```python
from build123d import *
from build123d.topology import SkipClean

# Parameters (mm, degrees)
BOSS_EXTRUDE1_DEPTH = 15
CUT_EXTRUDE1_DEPTH  = 5
BOSS_EXTRUDE2_DEPTH = 5
SKETCH3_R           = 15
CUT_EXTRUDE2_DEPTH  = 10


with BuildPart() as part:
    # Sketch1 → Boss-Extrude1 (new, symmetric)
    with BuildSketch(Plane.XY):
        with BuildLine():
            Line((-12.310096913, 2.170602221), (12.310096913, 2.170602221))
            ThreePointArc((12.310096913, 2.170602221), (0, -12.5), (-12.310096913, 2.170602221))
        make_face()
        with BuildLine():
            ThreePointArc((12.310096913, 2.170602221), (0, 12.5), (-12.310096913, 2.170602221))
            Line((-12.310096913, 2.170602221), (12.310096913, 2.170602221))
        make_face()
        with BuildLine():
            ThreePointArc((-12.310096913, 2.170602221), (0, -12.5), (12.310096913, 2.170602221))
            Line((12.310096913, 2.170602221), (15.337737359, -15))
            Line((15.337737359, -15), (-15.337737359, -15))
            Line((-15.337737359, -15), (-12.310096913, 2.170602221))
        make_face()
    extrude(amount=BOSS_EXTRUDE1_DEPTH, both=True)

    # Sketch1<3> → Cut-Extrude1 (cut, symmetric)
    with SkipClean():  # the faces are left unmerged after this step: merging them gives an invalid solid
        with BuildSketch(Plane.XY):
            with BuildLine():
                ThreePointArc((12.310096913, 2.170602221), (0, 12.5), (-12.310096913, 2.170602221))
                Line((-12.310096913, 2.170602221), (12.310096913, 2.170602221))
            make_face()
            with BuildLine():
                Line((-12.310096913, 2.170602221), (12.310096913, 2.170602221))
                ThreePointArc((12.310096913, 2.170602221), (0, -12.5), (-12.310096913, 2.170602221))
            make_face()
        extrude(amount=CUT_EXTRUDE1_DEPTH, both=True, mode=Mode.SUBTRACT)

    # Sketch2 → Boss-Extrude2 (add)
    with BuildSketch(Plane.XZ.offset(15)):
        with BuildLine():
            Line((-50, -7.5), (-23.848480035, -7.5))
            ThreePointArc((-23.848480035, -7.5), (-25, 0), (-23.848480035, 7.5))
            Line((-23.848480035, 7.5), (-50, 7.5))
            ThreePointArc((-50, 7.5), (-57.5, 0), (-50, -7.5))
        make_face()
        with BuildLine():
            Line((-23.848480035, -7.5), (-15.337737359, -7.5))
            Line((-15.337737359, -7.5), (-15.337737359, 7.5))
            Line((-15.337737359, 7.5), (-23.848480035, 7.5))
            ThreePointArc((-23.848480035, 7.5), (-25, 0), (-23.848480035, -7.5))
        make_face()
        with BuildLine():
            Line((-23.848480035, 7.5), (-15.337737359, 7.5))
            Line((-15.337737359, 7.5), (-15.337737359, 15))
            Line((-15.337737359, 15), (0, 15))
            Line((0, 15), (5.429049489, 24.403389552))
            ThreePointArc((5.429049489, 24.403389552), (-12.5, 21.650635095), (-23.848480035, 7.5))
        make_face()
        with BuildLine():
            ThreePointArc((5.429049489, 24.403389552), (12.5, 21.650635095), (18.419430546, 16.903389552))
            Line((18.419430546, 16.903389552), (31.495190528, 39.551270189))
            ThreePointArc((31.495190528, 39.551270189), (28.75, 49.796460718), (18.504809472, 47.051270189))
            Line((18.504809472, 47.051270189), (5.429049489, 24.403389552))
        make_face()
        with BuildLine():
            Line((15.337737359, 15), (15.337737359, 11.565740379))
            Line((15.337737359, 11.565740379), (18.419430546, 16.903389552))
            ThreePointArc((18.419430546, 16.903389552), (12.5, 21.650635095), (5.429049489, 24.403389552))
            Line((5.429049489, 24.403389552), (0, 15))
            Line((0, 15), (15.337737359, 15))
        make_face()
        with BuildLine():
            Line((18.419430546, 16.903389552), (15.337737359, 11.565740379))
            Line((15.337737359, 11.565740379), (15.337737359, -11.565740379))
            Line((15.337737359, -11.565740379), (18.419430546, -16.903389552))
            ThreePointArc((18.419430546, -16.903389552), (23.296842744, -9.069571003), (25, 0))
            ThreePointArc((25, 0), (23.296842744, 9.069571003), (18.419430546, 16.903389552))
        make_face()
        with BuildLine():
            ThreePointArc((6.495190528, -3.75), (3.75, -6.495190528), (0, -7.5))
            Line((0, -7.5), (-4.330127019, -7.5))
            Line((-4.330127019, -7.5), (0, -15))
            Line((0, -15), (15.337737359, -15))
            Line((15.337737359, -15), (15.337737359, -11.565740379))
            Line((15.337737359, -11.565740379), (8.660254038, 0))
            Line((8.660254038, 0), (6.495190528, -3.75))
        make_face()
        with BuildLine():
            Line((15.337737359, -15), (0, -15))
            Line((0, -15), (5.429049489, -24.403389552))
            ThreePointArc((5.429049489, -24.403389552), (12.5, -21.650635095), (18.419430546, -16.903389552))
            Line((18.419430546, -16.903389552), (15.337737359, -11.565740379))
            Line((15.337737359, -11.565740379), (15.337737359, -15))
        make_face()
        with BuildLine():
            ThreePointArc((18.419430546, -16.903389552), (12.5, -21.650635095), (5.429049489, -24.403389552))
            Line((5.429049489, -24.403389552), (18.504809472, -47.051270189))
            ThreePointArc((18.504809472, -47.051270189), (28.75, -49.796460718), (31.495190528, -39.551270189))
            Line((31.495190528, -39.551270189), (18.419430546, -16.903389552))
        make_face()
        with BuildLine():
            Line((-15.337737359, -15), (-15.337737359, -7.5))
            Line((-15.337737359, -7.5), (-23.848480035, -7.5))
            ThreePointArc((-23.848480035, -7.5), (-12.5, -21.650635095), (5.429049489, -24.403389552))
            Line((5.429049489, -24.403389552), (0, -15))
            Line((0, -15), (-15.337737359, -15))
        make_face()
        Polygon((0, -15), (-4.330127019, -7.5), (-15.337737359, -7.5), (-15.337737359, -15), align=None)
        with BuildLine():
            Line((-15.337737359, -7.5), (-4.330127019, -7.5))
            Line((-4.330127019, -7.5), (-6.495190528, -3.75))
            ThreePointArc((-6.495190528, -3.75), (-7.5, 0), (-6.495190528, 3.75))
            Line((-6.495190528, 3.75), (-4.330127019, 7.5))
            Line((-4.330127019, 7.5), (-15.337737359, 7.5))
            Line((-15.337737359, 7.5), (-15.337737359, -7.5))
        make_face()
        Polygon((-15.337737359, 15), (-15.337737359, 7.5), (-4.330127019, 7.5), (0, 15), align=None)
        with BuildLine():
            Line((6.495190528, 3.75), (8.660254038, 0))
            Line((8.660254038, 0), (15.337737359, 11.565740379))
            Line((15.337737359, 11.565740379), (15.337737359, 15))
            Line((15.337737359, 15), (0, 15))
            Line((0, 15), (-4.330127019, 7.5))
            Line((-4.330127019, 7.5), (0, 7.5))
            ThreePointArc((0, 7.5), (3.75, 6.495190528), (6.495190528, 3.75))
        make_face()
        Polygon((15.337737359, 11.565740379), (8.660254038, 0), (15.337737359, -11.565740379), align=None)
        with BuildLine():
            ThreePointArc((6.495190528, 3.75), (7.5, 0), (6.495190528, -3.75))
            Line((6.495190528, -3.75), (8.660254038, 0))
            Line((8.660254038, 0), (6.495190528, 3.75))
        make_face()
        with BuildLine():
            ThreePointArc((-6.495190528, -3.75), (-3.75, -6.495190528), (0, -7.5))
            ThreePointArc((0, -7.5), (3.75, -6.495190528), (6.495190528, -3.75))
            ThreePointArc((6.495190528, -3.75), (7.5, 0), (6.495190528, 3.75))
            ThreePointArc((6.495190528, 3.75), (3.75, 6.495190528), (0, 7.5))
            ThreePointArc((0, 7.5), (-3.75, 6.495190528), (-6.495190528, 3.75))
            ThreePointArc((-6.495190528, 3.75), (-7.5, 0), (-6.495190528, -3.75))
        make_face()
        with BuildLine():
            Line((-4.330127019, -7.5), (0, -7.5))
            ThreePointArc((0, -7.5), (-3.75, -6.495190528), (-6.495190528, -3.75))
            Line((-6.495190528, -3.75), (-4.330127019, -7.5))
        make_face()
        with BuildLine():
            Line((-4.330127019, 7.5), (-6.495190528, 3.75))
            ThreePointArc((-6.495190528, 3.75), (-3.75, 6.495190528), (0, 7.5))
            Line((0, 7.5), (-4.330127019, 7.5))
        make_face()
    extrude(amount=BOSS_EXTRUDE2_DEPTH)

    # Sketch3 → Cut-Extrude2 (cut)
    with BuildSketch(Plane.XY.offset(-5)):
        Circle(SKETCH3_R)
    extrude(amount=CUT_EXTRUDE2_DEPTH, mode=Mode.SUBTRACT)


solid = part.part
```
Work out the finished part from the listing and answer in its coordinate system (mm). A direction names the side the tool comes from. Coordinates: 2 decimals unless noted, no trailing zeros. Loops run counter-clockwise (first coordinate to the right, second up) from the corner with the lowest first, then second, coordinate; pieces in that order, holes last. Notation, with made-up numbers: (-33.5, 48.25) -> (-4.5, 48.25) arc R9 cw to (-4.5, 62.25) -> close; hole circle Ø5 at (-21.5, 61). An arc over 180 degrees is marked (long way). Answer as CSV lines item,"result".
Q1. Each of these flat-tipped pins is pushed along its axis until it touches: pin 1 (3 mm diameter, centred on y = -12.5, z = 12, fed in from +X); pin 2 (5.5 mm diameter, centred on x = -32, y = -17.5, fed in from -Z); pin 3 (4 mm diameter, centred on x = -12.5, y = -3, fed in from +Z). Where does it stop, or does it pass through?
Findings:
pin 1,"stops at x = 15.16"
pin 2,"stops at z = -7.5"
pin 3,"stops at z = 15"
Q2. A tool of negligible diameter and unlimited length cuts with its end or side. For faces 5 (the face through (0, -4, 15)), 6 (the face through (0, -1, 5)), 7 (the face through (-37, -17, -7.5)), 8 (the face through (28.892, -17.465, 49.712)), 9 (the face through (24.866, -17.465, 28.069)), from which of +Z, -Z, +X, -X, +Y, -Y can it reach the whole face along a straight path? Write none if from no direction.
Findings:
face 5,"+Z, +X, -X, +Y"
face 6,"+Y"
face 7,"-Z, -X, +Y, -Y"
face 8,"+Y, -Y"
face 9,"+X, +Y, -Y"
Q3. The part is cut by section B-B on y = 0.5. Write down the section's boundary in (x, z).
Findings:
outline,"(-12.6, -15) -> (12.6, -15) -> (12.6, -5) -> (-12.6, -5) -> close; (-12.6, 5) -> (12.6, 5) -> (12.6, 15) -> (-12.6, 15) -> close"
Q4. For a pull along Z with two mould halves and no side action, classify faces 1 (the face through (12.06, -17.46, 35.89)), 2 (the face through (0, -15, 0)), 3 (the face through (0.6, -15, 15.3)), 4 (the face through (0, -4, -15)) as +Z half, -Z half, draft (parallel to the pull), parting line (faces both ways), or undercut.
Findings:
face 1,"+Z half"
face 2,"undercut"
face 3,"draft"
face 4,"-Z half"
Q5. The part is cut by section C-C on x = 7. Write down the section's boundary in (y, z), and give its area (3 significant figures).
Findings:
outline,"(-20, -27.12) -> (-15, -27.12) -> (-15, -15) -> (10.36, -15) -> (10.36, -5) -> (-13.27, -5) -> (-13.27, 5) -> (10.36, 5) -> (10.36, 15) -> (-15, 15) -> (-15, 27.12) -> (-20, 27.12) -> close"
area,"796 mm²"
Q6. Find the intervals of material crossed by probe 1 along Z at (x, y) = (19.5, -16) (3 decimals); probe 2 along Y at (x, z) = (2.5, -17); probe 3 along Z at (x, y) = (-42.5, -17), in increasing order.
Findings:
probe 1,"z = -48.4 to -18.775, -15.644 to 15.644, 18.775 to 48.4"
probe 2,"y = -20 to -15"
probe 3,"z = -7.5 to 7.5"
Q7. The part is cut by section A-A on y = -13. Write down the section's boundary in (x, z).
Findings:
outline,"(-14.99, -15) -> (14.99, -15) -> (14.99, 15) -> (-14.99, 15) -> close; hole (-7.48, -5) -> (7.48, -5) -> (7.48, 5) -> (-7.48, 5) -> close"
Q8. The part is cut by section D-D on z = -11. Write down the section's boundary in (x, y), and give its area (3 significant figures).
Findings:
outline,"(-22.45, -20) -> (22.45, -20) -> (22.45, -15) -> (15.34, -15) -> (12.31, 2.17) arc R12.5 ccw to (-12.31, 2.17) -> (-15.34, -15) -> (-22.45, -15) -> close"
area,"891 mm²"
